Autodesk Inventor part; units mm, degrees
ref_plane "YZ Plane" through (0, 0, 0) normal (1, 0, 0) x (0, 1, 0)
ref_plane "XZ Plane" through (0, 0, 0) normal (0, 1, 0) x (-1, 0, 0)
ref_plane "XY Plane" through (0, 0, 0) normal (0, 0, 1) x (1, 0, 0)
sketch "Sketch1" plane through (0, 0, 0) normal (0, 0, 1) x (1, 0, 0)
  circle A0 centre (0, 0) radius 6.35
  circle A1 centre (0, 0) radius 2.3813
  circle A2 centre (0, 0) radius 3.5719
  circle A3 centre (0, 0) radius 5.1594
  dimension "d0" = 12.7
  dimension "d1" = 4.7625
  dimension "d2" = 7.1437
  dimension "d3" = 10.3187
extrude "Extrusion1" add sketch "Sketch1" along normal blind 2.4892
extrude "Extrusion2" add sketch "Sketch1" along normal blind 2.1082 contours A3
chamfer "Chamfer1" distance 0.254 angle 45 2 edges at (-6.35, 0, 2.4892) (-2.3813, 0, 2.4892)
mirror "Mirror1" about plane through (0, 0, 0) normal (0, 0, -1)
properties part number "R3-2RS"
Verification items for the finished model (mm, model axes). A direction names the side the tool comes from. Coordinates: 2 decimals unless noted, no trailing zeros. Write each loop counter-clockwise with the first axis right and the second up, starting at its lowest first coordinate (ties: lowest second). Pieces come first, ordered by that corner, then holes. Notation, with made-up numbers: (20.5, 48.5) - (33.5, 48.5) arc R25 ccw to (33.5, 60.5) - close; hole circle Ø9 at (77.25, 82). An arc over 180 degrees is marked (long way). One line per question, with ' | ' between items. Start each with the question number.
1. Material ranges on line 1 along Y through (x, z) = (0, -2.15); line 2 along Y through (x, z) = (0, 2.35); line 3 along Y through (x, z) = (0, 0.95), recorded low to high.
2. Gauge pin test, flat ends, axial feed: P1, Ø4, axis at x = 0, y = 0, coming from the -Z side; P2, Ø1, axis at x = 2.5, z = -2, coming from the -Y side. Record the tip position at first contact, or that the pin passes through.
3. Access from +Z, -Z, +X, -X, +Y, -Y to the whole of each face (thin tool, end or side, straight path). Record for faces 5 (the cylindrical face through (-3.8, -3.49, 2.3)), 6 (the flat face through (5, 3, -2.489)), 7 (the flat face through (-1, 4, -2.108)).
4. Section check C-C (z = 1.9). Enter the section's corners in (x, y), plus the area to 3 significant figures.
5. Draft check along Y on faces 1 (the cylindrical face through (-2.835, 2.173, 2.296)), 2 (the cylindrical face through (-1.38, 6.2, -0.03)), 3 (the flat face through (0, -3, -2.489)), 4 (the cylindrical face through (1.1, -2.11, 0.03)). Enter one of: released by +Y, released by -Y, zero draft, split by the parting line, or undercut.
Computed values:
1) line 1: -6.35 to -5.16, -3.57 to -2.38, 2.38 to 3.57, 5.16 to 6.35 | line 2: -6.24 to -5.16, -3.57 to -2.5, 2.5 to 3.57, 5.16 to 6.24 | line 3: -6.35 to -2.38, 2.38 to 6.35
2) P1: through | P2: y = -6.03
3) face 5: +Z | face 6: -Z, +X, -X, +Y, -Y | face 7: -Z
4) outline: circle Ø12.7 at (0, 0); hole circle Ø4.76 at (0, 0) | area: 109 mm²
5) face 1: undercut | face 2: split by the parting line | face 3: zero draft | face 4: undercut
